Check sheet for the drawn part. Datum: minimum x, y, z corner. Units: mm. A direction names the side the tool comes from. Round coordinates to 2 decimals unless told otherwise and drop trailing zeros. Write each loop counter-clockwise with the first axis right and the second up, starting at its lowest first coordinate (ties: lowest second). Pieces come first, ordered by that corner, then holes.
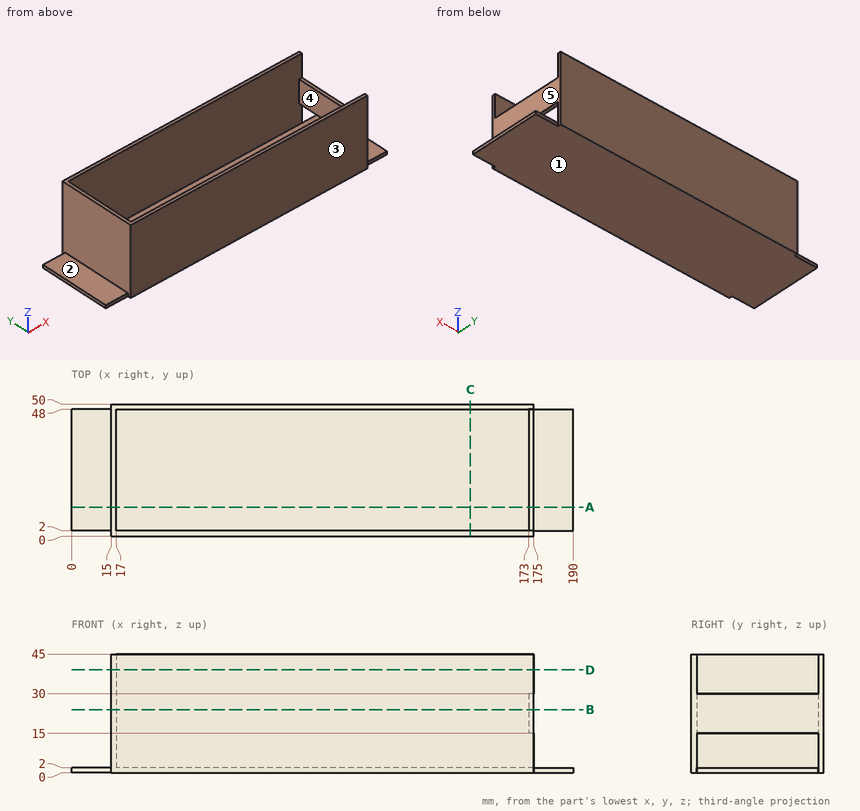
Q1. Sectioned sample at C-C (x = 151). Enter the section's corners in (y, z), plus the area to 3 significant figures.
Recorded:
outline: (0, 0) - (50, 0) - (50, 45) - (48, 45) - (48, 2) - (2, 2) - (2, 45) - (0, 45) - close
area: 272 mm2
Q2. Sectioned sample at D-D (z = 39). Enter the section's corners in (x, y).
Recorded:
outline: (15, 0) - (175, 0) - (175, 2) - (17, 2) - (17, 48) - (175, 48) - (175, 50) - (15, 50) - close
Q3. Material ranges on line 1 along Y through (x, z) = (105, 11.5); line 2 along X through (y, z) = (9.5, 28); line 3 along X through (y, z) = (18, 7), recorded low to high.
Recorded:
line 1: y = 0 to 2, 48 to 50
line 2: x = 15 to 17, 173 to 175
line 3: x = 15 to 17
Q4. Depth check by flat-ended pin: P1, Ø8, axis at y = 27, z = 23, coming from the +X side; P2, Ø1.5, axis at x = 116.5, y = 43.5, coming from the +Z side; P3, Ø1.6, axis at x = 10, z = 1, coming from the +Y side. Enter the tip coordinate at first touch or a pass-through.
Recorded:
P1: stops at x = 175
P2: stops at z = 2
P3: stops at y = 48
Q5. Release check for a two-part mould opening along X. For the marked faces 3, 4 and 5 record: released by +X, released by -X, zero draft, split by the parting line, or undercut.
Recorded:
face 3: zero draft
face 4: undercut
face 5: released by +X
Q6. Sectioned sample at A-A (y = 11). Enter the section's corners in (x, z), plus the area to 3 significant figures.
Recorded:
outline: (0, 0) - (190, 0) - (190, 2) - (17, 2) - (17, 45) - (15, 45) - (15, 2) - (0, 2) - close; (173, 15) - (175, 15) - (175, 30) - (173, 30) - close
area: 496 mm2
Q7. Sectioned sample at B-B (z = 24). Enter the section's corners in (x, y), plus the area to 3 significant figures.
Recorded:
outline: (15, 0) - (175, 0) - (175, 50) - (15, 50) - close; hole (17, 2) - (173, 2) - (173, 48) - (17, 48) - close
area: 824 mm2
Q8. Tool access check on the marked faces 1 and 2. Record the directions out of +Z, -Z, +X, -X, +Y, -Y that give a thin tool (end or side, any length) a straight path to the whole face; none if there is none.
Recorded:
face 1: -Z, +X, -X, +Y, -Y
face 2: +Z, -X, +Y, -Y
